Input: dimensioned drawing with shaded views. Units: mm. Origin: part minimum x, y, z. A direction names the side the tool comes from. Round coordinates to 2 decimals unless told otherwise and drop trailing zeros. Loops run counter-clockwise (first coordinate to the right, second up) from the corner with the lowest first, then second, coordinate; pieces in that order, holes last. Notation, with made-up numbers: (78, -34.75) - (124, -34.75) arc R15 ccw to (124, -15.75) - close; hole circle Ø8 at (58.25, -11). An arc over 180 degrees is marked (long way). One line per question, with ' | ' between items. Start each with the question number.
Item 1: Section C-C, the plane y = 2.25. Return loops of the section in (x, z), plus the area to 3 significant figures.
Item 2: Set-up query: the marked faces 1 and 2. Return all of +Z, -Z, +X, -X, +Y, -Y with unobstructed straight access to the full face (end or side cutting, diameter ignored); none if empty.
Item 3: Material intervals for line 1 along Z through (x, y) = (3, 6.5); line 2 along Y through (x, z) = (6, 34) (1 decimal); line 3 along Z through (x, y) = (2.75, 5.25), sorted ascending.
Item 4: First-contact query: pin 1 (1.6 mm diameter, centred on y = 0.5, z = 35, fed in from +X); pin 2 (0.7 mm diameter, centred on y = 9, z = 35, fed in from +X); pin 3 (1.5 mm diameter, centred on x = 7.5, y = 1.5, fed in from +Z). Flat tips, straight axial feed; report the tip coordinate or a pass-through.
Item 5: Section D-D, the plane z = 28.5. Return loops of the section in (x, y) (1 decimal).
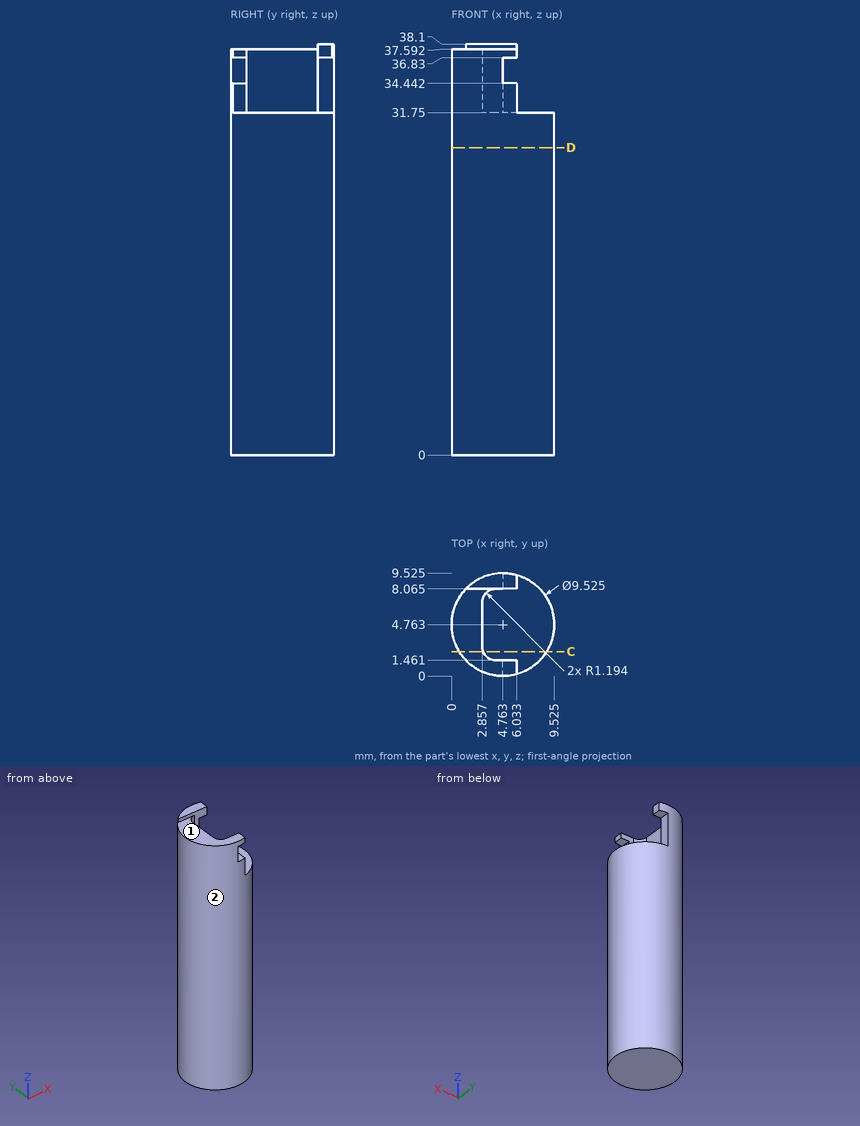
Return value:
1) outline: (0.72, 0) - (8.81, 0) - (8.81, 31.75) - (2.93, 31.75) - (2.93, 37.59) - (0.72, 37.59) - close | area: 270 mm2
2) face 1: +Z, +X, -X, -Y | face 2: +Z, -Z
3) line 1: 0 to 31.75 | line 2: 0.2 to 1.5 | line 3: 0 to 37.59
4) pin 1: x = 6.03 | pin 2: x = 4.76 | pin 3: z = 31.75
5) outline: circle Ø9.5 at (4.8, 4.8)
